```python
from build123d import *

# Parameters (mm, degrees)
F0_W     = 57
F0_H     = 28
F1_DEPTH = 16
F2_T     = -1
F3_W     = 20.5
F3_H     = 2.5
F4_DEPTH = 3
F5_W     = 8.5
F5_H     = 3.5
F6_DEPTH = 3


with BuildPart() as f1:
    # F0 (on Top) → F1 (new body)
    with BuildSketch(Plane.XY):
        Rectangle(F0_W, F0_H)
    extrude(amount=F1_DEPTH)

    # F2
    f2_openings = [f1.faces().sort_by_distance(p)[0] for p in [
        (0, 0, 16),
    ]]
    offset(amount=F2_T, openings=f2_openings)

    # F3 (on face) → F4 (cut)
    with BuildSketch(Plane.XZ.offset(14)):
        with Locations((4.25, 12.55)):
            Rectangle(F3_W, F3_H)
    extrude(amount=-F4_DEPTH, mode=Mode.SUBTRACT)

    # F5 (on face) → F6 (cut)
    with BuildSketch(Plane.YZ.offset(28.5)):
        with Locations((1.25, 3.25)):
            Rectangle(F5_W, F5_H)
    extrude(amount=-F6_DEPTH, mode=Mode.SUBTRACT)


solid = f1.part
```
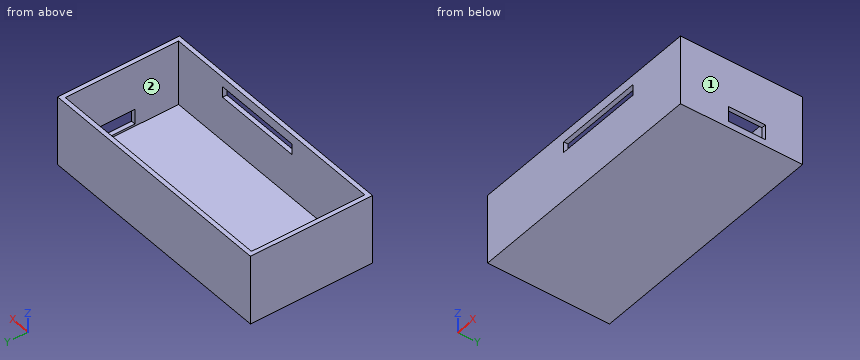
CAD build for the part. Positions are in the model's coordinates, mm. Face numbers are marked on the shaded views. A direction names the side the tool comes from. Give positions to 0.01 mm unless a question says otherwise; leave off trailing zeros. Loops run counter-clockwise (first coordinate to the right, second up) from the corner with the lowest first, then second, coordinate; pieces in that order, holes last. Notation, with made-up numbers: (-9.75, 48) - (11.25, 48) arc R24 cw to (11.25, 76) - close; hole circle Ø8 at (-17, 20). An arc over 180 degrees is marked (long way). Put each result on its own line as item: value.
Q1. Probe line 1 along X through (y, z) = (6, 8); line 2 along Y through (x, z) = (-20, 14); line 3 along Z through (x, y) = (-23.5, -3.75). List the from-to ranges inside material, lowest first.
Filled in:
line 1: x = -28.5 to -27.5, 27.5 to 28.5
line 2: y = -14 to -13, 13 to 14
line 3: z = 0 to 1
Q2. Flat gauge pin, fed straight in: pin 1 (1.5 mm diameter, centred on x = 18, y = -7.5, fed in from +Z). Where does the tip first touch, or does it go through?
Filled in:
pin 1: stops at z = 1
Q3. Slice it at B-B (y = 0.25). Give the cut face in (x, z).
Filled in:
outline: (-28.5, 0) - (28.5, 0) - (28.5, 1.5) - (27.5, 1.5) - (27.5, 1) - (-27.5, 1) - (-27.5, 16) - (-28.5, 16) - close; (27.5, 5) - (28.5, 5) - (28.5, 16) - (27.5, 16) - close
Q4. Slice it at A-A (x = -5). Give the cut face in (y, z).
Filled in:
outline: (-14, 0) - (14, 0) - (14, 16) - (13, 16) - (13, 1) - (-13, 1) - (-13, 11.3) - (-14, 11.3) - close; (-14, 13.8) - (-13, 13.8) - (-13, 16) - (-14, 16) - close
Q5. Slice it at C-C (z = 6.5). Give the cut face in (x, y).
Filled in:
outline: (-28.5, -14) - (28.5, -14) - (28.5, 14) - (-28.5, 14) - close; hole (-27.5, -13) - (27.5, -13) - (27.5, 13) - (-27.5, 13) - close
Q6. Slice it at D-D (z = 3.75). Give the cut face in (x, y).
Filled in:
outline: (-28.5, -14) - (28.5, -14) - (28.5, -3) - (27.5, -3) - (27.5, -13) - (-27.5, -13) - (-27.5, 13) - (27.5, 13) - (27.5, 5.5) - (28.5, 5.5) - (28.5, 14) - (-28.5, 14) - close
Q7. Tool access for the marked faces 1 and 2: list every direction of +Z, -Z, +X, -X, +Y, -Y with a clear straight run to the whole face (end or side of a thin tool).
Filled in:
face 1: +Z, -Z, +X, +Y, -Y
face 2: +Z
